Input: part model. Units: mm. Frame: model coordinates. Face numbers are marked on the shaded views. Give positions to 0.01 mm unless a question says otherwise; leave off trailing zeros. Loops run counter-clockwise (first coordinate to the right, second up) from the corner with the lowest first, then second, coordinate; pieces in that order, holes last. Notation, with made-up numbers: (67.5, 28) -> (81.5, 28) arc R20 ccw to (81.5, 62) -> close; hole circle Ø10 at (4.25, 46). An arc over 180 degrees is marked (long way). One line per question, with ' | ' between items.
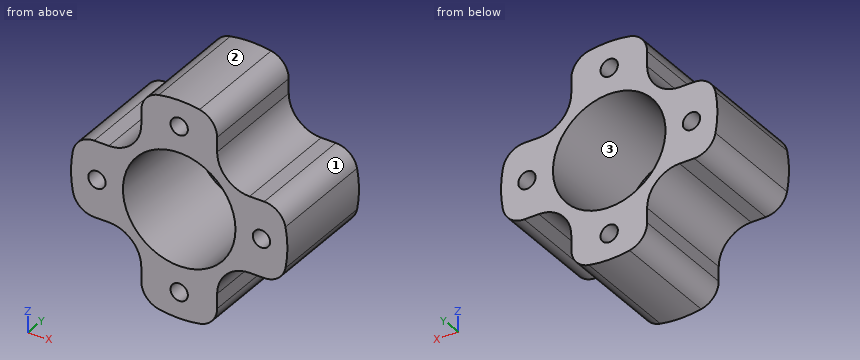
from build123d import *

# Parameters (mm, degrees)
F0_R     = 25
F0_R_2   = 2
F1_DEPTH = 25
F3_DEPTH = 25.001
F4_R     = 5
F5_R     = 13
F6_DEPTH = 25.001


with BuildPart() as f1:
    # F0 (on Front) → F1 (new body)
    with BuildSketch(Plane.XZ):
        Circle(F0_R)
        with Locations((0, -19)):
            Circle(F0_R_2, mode=Mode.SUBTRACT)
        with Locations((-19, 0)):
            Circle(F0_R_2, mode=Mode.SUBTRACT)
        with Locations((19, 0)):
            Circle(F0_R_2, mode=Mode.SUBTRACT)
        with Locations((0, 19)):
            Circle(F0_R_2, mode=Mode.SUBTRACT)
    extrude(amount=F1_DEPTH)

    # F2 (on Front) → F3 (cut, through all)
    with BuildSketch(Plane.XZ):
        with BuildLine():
            Line((-23.7634559673, 8.7634559673), (-16.2634559673, 8.7634559673))
            ThreePointArc((-16.2634559673, 8.7634559673), (-10.9601551084, 10.9601551084), (-8.7634559673, 16.2634559673))
            Line((-8.7634559673, 16.2634559673), (-8.7634559673, 23.7634559673))
            Line((-8.7634559673, 23.7634559673), (-23.7634559673, 23.7634559673))
            Line((-23.7634559673, 23.7634559673), (-23.7634559673, 8.7634559673))
        make_face()
        with BuildLine():
            Line((8.7634559673, 23.7634559673), (8.7634559673, 16.2634559673))
            ThreePointArc((8.7634559673, 16.2634559673), (10.9601551084, 10.9601551084), (16.2634559673, 8.7634559673))
            Line((16.2634559673, 8.7634559673), (23.7634559673, 8.7634559673))
            Line((23.7634559673, 8.7634559673), (23.7634559673, 23.7634559673))
            Line((23.7634559673, 23.7634559673), (8.7634559673, 23.7634559673))
        make_face()
        with BuildLine():
            ThreePointArc((-8.7634559673, -16.2634559673), (-10.9601551084, -10.9601551084), (-16.2634559673, -8.7634559673))
            Line((-16.2634559673, -8.7634559673), (-23.7634559673, -8.7634559673))
            Line((-23.7634559673, -8.7634559673), (-23.7634559673, -23.7634559673))
            Line((-23.7634559673, -23.7634559673), (-8.7634559673, -23.7634559673))
            Line((-8.7634559673, -23.7634559673), (-8.7634559673, -16.2634559673))
        make_face()
        with BuildLine():
            ThreePointArc((16.2634559673, -8.7634559673), (10.9601551084, -10.9601551084), (8.7634559673, -16.2634559673))
            Line((8.7634559673, -16.2634559673), (8.7634559673, -23.7634559673))
            Line((8.7634559673, -23.7634559673), (23.7634559673, -23.7634559673))
            Line((23.7634559673, -23.7634559673), (23.7634559673, -8.7634559673))
            Line((23.7634559673, -8.7634559673), (16.2634559673, -8.7634559673))
        make_face()
    extrude(amount=F3_DEPTH, mode=Mode.SUBTRACT)

    # F4
    f4_edges = [f1.edges().sort_by_distance(p)[0] for p in [
        (8.763456, -12.5, 23.413711),
        (-8.763456, -12.5, 23.413711),
        (-23.413711, -12.5, 8.763456),
        (-23.413711, -12.5, -8.763456),
        (-8.763456, -12.5, -23.413711),
        (8.763456, -12.5, -23.413711),
        (23.413711, -12.5, -8.763456),
        (23.413711, -12.5, 8.763456),
    ]]
    fillet(f4_edges, radius=F4_R)

    # F5 (on Front) → F6 (cut, through all)
    with BuildSketch(Plane.XZ):
        Circle(F5_R)
    extrude(amount=F6_DEPTH, mode=Mode.SUBTRACT)


solid = f1.part
1. Section query B-B (z = -19). Output: boundary loops of the cut face in (x, y), then the cut area to 3 significant figures.
Determined:
outline: (-8.76, -25) -> (-2, -25) -> (-2, 0) -> (-8.76, 0) -> close; (2, -25) -> (8.76, -25) -> (8.76, 0) -> (2, 0) -> close | area: 338 mm2
2. Section query D-D (x = 0). Output: boundary loops of the cut face in (y, z), then the cut area to 3 significant figures.
Determined:
outline: (-25, -25) -> (0, -25) -> (0, -21) -> (-25, -21) -> close; (-25, -17) -> (0, -17) -> (0, -13) -> (-25, -13) -> close; (-25, 13) -> (0, 13) -> (0, 17) -> (-25, 17) -> close; (-25, 21) -> (0, 21) -> (0, 25) -> (-25, 25) -> close | area: 400 mm2
3. Pull-direction query (X, two-part tool) for the marked faces 1, 2 and 3; classes: pulls with the +X half, pulls with the -X half, needs draft (parallel to the pull), parting line crosses it, or undercut.
Determined:
face 1: pulls with the +X half | face 2: parting line crosses it | face 3: undercut
4. Section query C-C (y = -17.5). Count the separate pieces of the cut face and the enclosed holes in it, then the cut area to 3 significant figures.
Determined:
separate pieces: 1 | enclosed holes: 5 | area: 853 mm2
5. Pin query (flat end, axial travel): P1, Ø3, axis at y = -11.5, z = -4.5, coming from the -X side; P2, Ø2, axis at y = -12, z = 12, coming from the -X side; P3, Ø1, axis at y = -15, z = 18, coming from the -X side. Return the tip coordinate at first contact, or that it passes through.
Determined:
P1: stops at x = -24.82 | P2: stops at x = -10.92 | P3: stops at x = -8.76
6. Section query A-A (x = -19). Output: boundary loops of the cut face in (y, z).
Determined:
outline: (-25, -8.76) -> (0, -8.76) -> (0, -2) -> (-25, -2) -> close; (-25, 2) -> (0, 2) -> (0, 8.76) -> (-25, 8.76) -> close
7. Ray query, line 1 along Z through (x, y) = (0, -14.75); line 2 along Z through (x, y) = (-19, -19.75); line 3 along X through (y, z) = (-13.25, 16.5). Return the intervals inside material, ascending. Write a range as from..to.
Determined:
line 1: z = -25..-21, -17..-13, 13..17, 21..25 | line 2: z = -8.76..-2, 2..8.76 | line 3: x = -8.76..8.76
